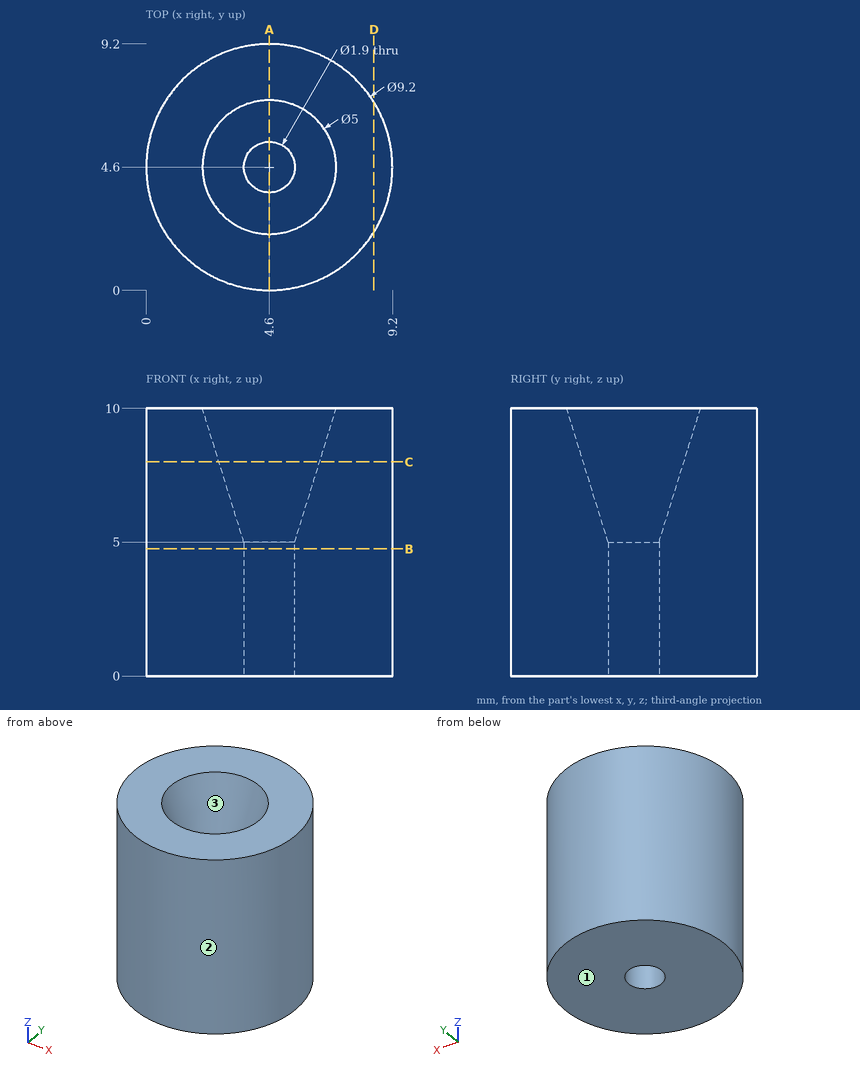
Verification items for this drawing (mm, ordinates from the low corner). Round coordinates to 2 decimals unless told otherwise and drop trailing zeros. Loops run counter-clockwise (first coordinate to the right, second up) from the corner with the lowest first, then second, coordinate; pieces in that order, holes last. Notation, with made-up numbers: M -13.5,11.5 L -3.5,11.5 A32 cw -3.5,48.5 Z; hole C 3.5,56 d2. An arc over 180 degrees is marked long. Answer as a JSON object with one key per item and string values.
1. Scan lines: line 1 (Y direction, x = 4.6, z = 2.4); line 2 (X direction, y = 5, z = 8); line 3 (Y direction, x = 3.75, z = 8.5). Record each from-to range of solid material in increasing order.
Reply:
{"line 1": "y = 0 to 3.65, 5.55 to 9.2", "line 2": "x = 0.02 to 2.76, 6.44 to 9.18", "line 3": "y = 0.08 to 2.75, 6.45 to 9.12"}
2. Section check A-A (x = 4.6). Record the boundary of the cut face in (y, z), plus the area to 4 significant figures.
Reply:
{"outline": "M 0,0 L 3.65,0 L 3.65,5 L 2.1,10 L 0,10 Z; M 5.55,0 L 9.2,0 L 9.2,10 L 7.1,10 L 5.55,5 Z", "area": "65.25 mm²"}
3. Section check B-B (z = 4.75). Record the boundary of the cut face in (x, y).
Reply:
{"outline": "C 4.6,4.6 d9.2; hole C 4.6,4.6 d1.9"}
4. Gauge pin test, flat ends, axial feed: P1, Ø1.5, axis at y = 1, z = 3, coming from the -X side; P2, Ø2, axis at x = 1, z = 7.5, coming from the +Y side; P3, Ø1.5, axis at y = 3, z = 7.5, coming from the +X side. Record the tip position at first contact, or that the pin passes through.
Reply:
{"P1": "stops at x = 0.99", "P2": "stops at y = 8.39", "P3": "stops at x = 9.12"}
5. Mould release check, pull along Y, two halves, no side actions. Record for the marked faces 1, 2 and 3: pulls with the +Y half, pulls with the -Y half, needs draft (parallel to the pull), parting line crosses it, or undercut.
Reply:
{"face 1": "needs draft", "face 2": "parting line crosses it", "face 3": "undercut"}
6. Section check C-C (z = 8). Record the boundary of the cut face in (x, y).
Reply:
{"outline": "C 4.6,4.6 d9.2; hole C 4.6,4.6 d3.76"}
7. Section check D-D (x = 8.5). Record the boundary of the cut face in (y, z).
Reply:
{"outline": "M 2.16,0 L 7.04,0 L 7.04,10 L 2.16,10 Z"}
